Source: CAD feature listing. Evaluate the final solid. Frame: model axes, mm. A direction names the side the tool comes from. Coordinates: 2 decimals unless noted, no trailing zeros. Write each loop counter-clockwise with the first axis right and the second up, starting at its lowest first coordinate (ties: lowest second). Pieces come first, ordered by that corner, then holes. Notation, with made-up numbers: (20, 67) - (55, 67) arc R21 ccw to (55, 95) - close; hole circle Ø6 at (-32.5, -21). An arc over 180 degrees is marked (long way). One line per question, with ' | ' between items.
from build123d import *

# Parameters (mm, degrees)
SKETCH1_W           = 12
SKETCH1_H           = 12
BOSS_EXTRUDE1_DEPTH = 11
SHELL1_T            = -2
SKETCH3_R           = 0.625
CUT_EXTRUDE1_DEPTH  = 10


with BuildPart() as part:
    # Sketch1 → Boss-Extrude1 (new body)
    with BuildSketch(Plane(origin=(0, 0, 0), x_dir=(1, 0, 0), z_dir=(0, 1, 0))):
        with Locations((6, 6)):
            Rectangle(SKETCH1_W, SKETCH1_H)
    extrude(amount=BOSS_EXTRUDE1_DEPTH)

    # Shell1
    shell1_openings = [part.faces().sort_by_distance(p)[0] for p in [
        (6, 11, -6),
    ]]
    offset(amount=SHELL1_T, openings=shell1_openings, kind=Kind.INTERSECTION)

    # Sketch3 → Cut-Extrude1 (cut)
    with BuildSketch(Plane.XZ):
        with Locations((6, -4.73)):
            Circle(SKETCH3_R)
        with Locations((6, -7.27)):
            Circle(SKETCH3_R)
    extrude(amount=-CUT_EXTRUDE1_DEPTH, mode=Mode.SUBTRACT)


solid = part.part
Item 1: Ray query, line 1 along Z through (x, y) = (6, 0.45) (3 decimals); line 2 along X through (y, z) = (5.75, -2.5); line 3 along Z through (x, y) = (6.25, 6.25). Return the intervals inside material, ascending. Write a range as [from, to].
Check sheet entries:
line 1: [-12, -7.895], [-6.645, -5.355], [-4.105, 0] | line 2: [0, 2], [10, 12] | line 3: [-12, -10], [-2, 0]
Item 2: Access query for faces 4 (the face through (5.92, 0.99, -4.11)), 5 (the face through (6, 2, -6)). Directions: +Z, -Z, +X, -X, +Y, -Y. A direction counts if a zero-diameter tool reaches every point of the face in a straight line with its end or side. Return the directions, or none.
Check sheet entries:
face 4: +Y, -Y | face 5: +Y
Item 3: Mould query, pull axis X, two halves, no side actions, for faces 1 (the face through (6, 5, -12)), 2 (the face through (0, 5, -6)), 3 (the face through (6, 6, -10)). Classes: pulls with the +X half, pulls with the -X half, needs draft (parallel to the pull), parting line crosses it, or undercut.
Check sheet entries:
face 1: needs draft | face 2: pulls with the -X half | face 3: undercut
Item 4: Cut plane B-B on x = 6. Return loops of the section in (y, z) (3 decimals), and give its area (3 significant figures).
Check sheet entries:
outline: (0, -12) - (11, -12) - (11, -10) - (2, -10) - (2, -7.895) - (0, -7.895) - close; (0, -6.645) - (2, -6.645) - (2, -5.355) - (0, -5.355) - close; (0, -4.105) - (2, -4.105) - (2, -2) - (11, -2) - (11, 0) - (0, 0) - close | area: 55.0 mm²
Item 5: Cut plane A-A on z = -7.27. Return loops of the section in (x, y) (3 decimals).
Check sheet entries:
outline: (0, 0) - (5.375, 0) - (5.375, 2) - (2, 2) - (2, 11) - (0, 11) - close; (6.625, 0) - (12, 0) - (12, 11) - (10, 11) - (10, 2) - (6.625, 2) - close
Item 6: Cut plane C-C on y = 3. Return loops of the section in (x, z), and give its area (3 significant figures).
Check sheet entries:
outline: (0, -12) - (12, -12) - (12, 0) - (0, 0) - close; hole (2, -10) - (10, -10) - (10, -2) - (2, -2) - close | area: 80.0 mm²
Item 7: Cut plane D-D on z = -2.5. Return loops of the section in (x, y), and give its area (3 significant figures).
Check sheet entries:
outline: (0, 0) - (12, 0) - (12, 11) - (10, 11) - (10, 2) - (2, 2) - (2, 11) - (0, 11) - close | area: 60.0 mm²
